Autodesk Inventor part; units mm, degrees
ref_plane "YZ Plane" through (0, 0, 0) normal (1, 0, 0) x (0, 1, 0)
ref_plane "XZ Plane" through (0, 0, 0) normal (0, 1, 0) x (-1, 0, 0)
ref_plane "XY Plane" through (0, 0, 0) normal (0, 0, 1) x (1, 0, 0)
sketch "Sketch1" plane through (0, 0, 0) normal (1, 0, 0) x (0, 1, 0)
  line L0 (-44.45, -25.4) -> (44.45, -25.4)
  line L1 (44.45, -25.4) -> (44.45, 25.4)
  line L2 (44.45, 25.4) -> (-44.45, 25.4)
  line L3 (-44.45, 25.4) -> (-44.45, -25.4)
  line L4 (-44.45, -25.4) -> (44.45, 25.4) construction
  line L5 (44.45, -25.4) -> (-44.45, 25.4) construction
  point P0 (0, 0)
  dimension "d0" = 88.9
  dimension "d1" = 50.8
extrude "Extrusion1" add sketch "Sketch1" along normal blind 6.35
sketch "Sketch2" plane through (6.35, 0, 0) normal (1, 0, 0) x (0, 0, -1)
  line L0 (12.7, -36.4998) -> (-12.7, -36.4998) construction
  line L1 (-12.7, -36.4998) -> (-12.7, -1.5748) construction
  line L2 (-12.7, -1.5748) -> (12.7, -1.5748) construction
  line L3 (12.7, -1.5748) -> (12.7, -36.4998) construction
  line L4 (12.7, -36.4998) -> (-12.7, -1.5748) construction
  line L5 (-12.7, -36.4998) -> (12.7, -1.5748) construction
  line L6 (-25.4, -44.45) -> (25.4, -44.45) construction
  line L7 (25.4, 44.45) -> (-25.4, 44.45) construction
  line L8 (25.4, -44.45) -> (25.4, 44.45) construction
  point P0 (0, 0)
  point P1 (0, -19.0373)
  point P2 (15.875, 38.1)
  point P3 (15.875, 25.4)
  point P4 (0, 44.45)
  point P5 (0, 44.45)
  dimension "d4" = 25.4
  dimension "d5" = 34.925
  dimension "d6" = 7.9502
  dimension "d7" = 12.7
  dimension "d23" = 6.35
  dimension "d24" = 9.525
hole "Hole1" at (6.35, -36.4998, 12.7) at (6.35, -36.4998, -12.7) at (6.35, -1.5748, -12.7) at (6.35, -1.5748, 12.7) direction (-1, 0, 0) diameter 3.9624 end through all
hole "Hole2" at (6.35, 38.1, -15.875) at (6.35, 25.4, -15.875) direction (-1, 0, 0) diameter 5.1054 end through all
properties part number "EL2-027" material "Aluminum 6061"
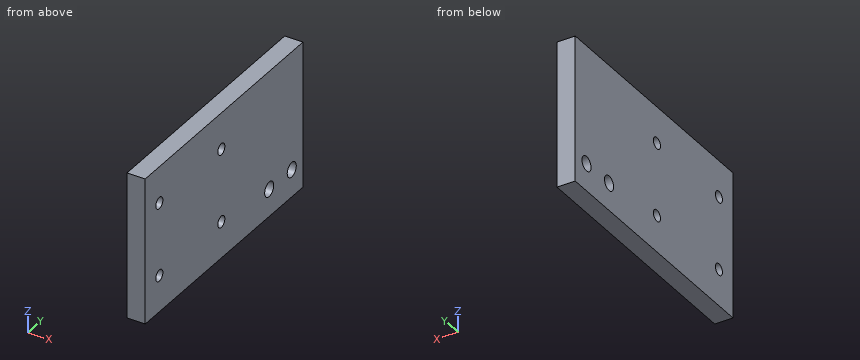
For this review, take the finished solid that the model builds, in its own axes (mm). Give positions to 0.01 mm unless a question says otherwise; leave off trailing zeros. Loops run counter-clockwise (first coordinate to the right, second up) from the corner with the lowest first, then second, coordinate; pieces in that order, holes last. Notation, with made-up numbers: M 4,32.5 L 51,32.5 A9 ccw 51,40.5 Z; hole C 42,57.25 d5. An arc over 180 degrees is marked long. Put each result on its own line as item: value. Start each with the question number.
(1) Add section A-A, the plane y = 38.1. Write out the cut boundary in (x, z).
(2) Wall thickness on L1, parallel to Y at x = 1.75, z = -12.7; L2, parallel to Z at x = 5, y = -1.5; L3, parallel to Y at x = 2, z = 13: over which ranges is each line inside the solid? List them lowest first.
(3) For pin 1 (3 mm diameter, centred on y = -1.57, z = -12.7, fed in from -X), flat-tipped, find the tip position at first contact; note if it passes through.
(4) Add section B-B, the plane z = 12.7. Write out the cut boundary in (x, y), then the cut area to 3 significant figures.
(5) Add section C-C, the plane x = 3.5. Write out the cut boundary in (y, z) (3 decimals), then the cut area to 3 significant figures.
Result:
1. outline: M 0,-25.4 L 6.35,-25.4 L 6.35,-18.43 L 0,-18.43 Z; M 0,-13.32 L 6.35,-13.32 L 6.35,25.4 L 0,25.4 Z
2. L1: y = -44.45 to -38.48, -34.52 to -3.56, 0.41 to 44.45
2. L2: z = -25.4 to -14.68, -10.72 to 10.72, 14.68 to 25.4
2. L3: y = -44.45 to -38.46, -34.54 to -3.53, 0.38 to 44.45
3. pin 1: passes through
4. outline: M 0,-44.45 L 6.35,-44.45 L 6.35,-38.48 L 0,-38.48 Z; M 0,-34.52 L 6.35,-34.52 L 6.35,-3.56 L 0,-3.56 Z; M 0,0.41 L 6.35,0.41 L 6.35,44.45 L 0,44.45 Z
4. area: 514 mm^2
5. outline: M -44.45,-25.4 L 44.45,-25.4 L 44.45,25.4 L -44.45,25.4 Z; hole C -36.5,-12.7 d3.962; hole C -36.5,12.7 d3.962; hole C -1.575,-12.7 d3.962; hole C -1.575,12.7 d3.962; hole C 25.4,-15.875 d5.105; hole C 38.1,-15.875 d5.105
5. area: 4,430 mm^2
